```python
from build123d import *

# Parameters (mm, degrees)
RESSALTO_EXTRUS_O1_DEPTH        = 7.5
FURO_ROSCADO_DE_M31_D           = 2.5
FURO_ROSCADO_DE_M31_DEPTH       = 7.5
FURO_ROSCADO_DE_M31_CSINK_D     = 3.05
FURO_ROSCADO_DE_M31_CSINK_ANGLE = 90
FURO_ROSCADO_DE_M31_TIP         = 0.751075774
CHANFRO1_SIZE                   = 5


with BuildPart() as part:
    # Esboço1 → Ressalto-extrusão1 (new, symmetric)
    with BuildSketch(Plane(origin=(0, 0, 0), x_dir=(1, 0, 0), z_dir=(0, 1, 0))):
        Polygon((3.666174209, 6.35), (-3.666174209, 6.35), (-8, 6.35), (-8, -6.35), (8, -6.35), (8, 6.35), align=None)
    extrude(amount=RESSALTO_EXTRUS_O1_DEPTH, both=True)

    # Esboço5 → Furo roscado de M81 (revolve, cut)
    with BuildSketch(Plane(origin=(0, 7.5, 0), x_dir=(0, 0, 1), z_dir=(1, 0, 0))):
        Polygon((0, 0), (0, 15), (4, 15), (3.4, 14.4), (3.4, 0.6), (4, 0), align=None)
    revolve(axis=Axis((0, 13.85, 0), (0, -1, 0)), mode=Mode.SUBTRACT)

    # Furo roscado de M31
    with Locations(Plane(origin=(0, 0, -6.35), x_dir=(-1, 0, 0), z_dir=(0, 0, -1))):
        with Locations((-6, 0), (6, 0)):
            CounterSinkHole(FURO_ROSCADO_DE_M31_D / 2, FURO_ROSCADO_DE_M31_CSINK_D / 2, depth=FURO_ROSCADO_DE_M31_DEPTH, counter_sink_angle=FURO_ROSCADO_DE_M31_CSINK_ANGLE)
            with Locations((0, 0, -(FURO_ROSCADO_DE_M31_DEPTH + FURO_ROSCADO_DE_M31_TIP / 2))):  # 118° drill point
                Cone(0, FURO_ROSCADO_DE_M31_D / 2, FURO_ROSCADO_DE_M31_TIP, mode=Mode.SUBTRACT)

    # Chanfro1
    chanfro1_edges = [part.edges().sort_by_distance(p)[0] for p in [
        (8, 0, 6.35),
        (-8, 0, 6.35),
    ]]
    chamfer(chanfro1_edges, length=CHANFRO1_SIZE)


solid = part.part
```
Here's how the part is built. I have some questions about the finished solid (model axes, mm). A direction names the side the tool comes from. Round coordinates to 2 decimals unless told otherwise and drop trailing zeros. Order: outer loops, then holes, each group sorted by start corner. A loop starts at its lowest first (then second) coordinate and runs counter-clockwise, first axis right, second up. Notation, with made-up numbers: (-24.75, 79.5) -> (-3.75, 79.5) arc R26 ccw to (-3.75, 116.5) -> close; hole circle Ø3 at (-24.75, 7.5). An arc over 180 degrees is marked (long way). Use a Markdown table: item, result. Add a question column.
(1) For pin 1 Ø3 at (x, y) = (-6, 0) entering from -Z (3 decimals); pin 2 Ø2 at (x, y) = (6, 0) entering from +Z, each with a flat end and sliding along its axis, tell me the tip position at first contact or that it passes through.
(2) I need wall thicknesses on line 1 along Z through (x, y) = (0, -3); line 2 along X through (y, z) = (1.75, 0); line 3 along X through (y, z) = (0, -0.75). Which ranges of each line are inside material? Lowest first, please.
(3) For faces 1 (the face through (-7.25, 0.05, -2.41)), 2 (the face through (-0.1, -7.5, -4.3)), which set-ups out of +Z, -Z, +X, -X, +Y, -Y let a thin tool reach every point of the face, with its end or its side?
(4) Suppose I cut it at C-C, the plane x = 0. Please give me the cut outline in (y, z), and give its area (3 significant figures).
(5) Suppose I cut it at A-A, the plane z = 0. Please give me the cut outline in (x, y).
(6) If we mould it in two halves opening along Z, with no side actions, what happens to faces 3 (the face through (-0.1, 7.5, -4.3)), 4 (the face through (-5.78, 0.01, 1.77)), 5 (the face through (3.32, 0.1, -0.74)), 6 (the face through (-5.465, -0.105, 3.885))? For each: released by +Z, released by -Z, zero draft, split by the parting line, or undercut.
(7) Suppose I cut it at D-D, the plane z = -4.5. Please give me the cut outline in (x, y), and give its area (3 significant figures).
(8) Suppose I cut it at B-B, the plane y = -6. Please give me the cut outline in (x, z), and give its area (3 significant figures).
Verdict:
| question | item | result |
|---|---|---|
| 1 | pin 1 | z = -6.325 |
| 1 | pin 2 | z = 4.35 |
| 2 | line 1 | -6.35 to -3.4, 3.4 to 6.35 |
| 2 | line 2 | -8 to -3.4, 3.4 to 8 |
| 2 | line 3 | -8 to -7.25, -4.75 to -3.32, 3.32 to 4.75, 7.25 to 8 |
| 3 | face 1 | -Z |
| 3 | face 2 | +Z, -Z, +X, -X, -Y |
| 4 | outline | (-7.5, -6.35) -> (7.5, -6.35) -> (7.5, -4) -> (6.9, -3.4) -> (-6.9, -3.4) -> (-7.5, -4) -> close; (-7.5, 4) -> (-6.9, 3.4) -> (6.9, 3.4) -> (7.5, 4) -> (7.5, 6.35) -> (-7.5, 6.35) -> close |
| 4 | area | 87.8 mm2 |
| 5 | outline | (-8, -7.5) -> (-4, -7.5) -> (-3.4, -6.9) -> (-3.4, 6.9) -> (-4, 7.5) -> (-8, 7.5) -> close; (3.4, -6.9) -> (4, -7.5) -> (8, -7.5) -> (8, 7.5) -> (4, 7.5) -> (3.4, 6.9) -> close; hole circle Ø2.5 at (-6, 0); hole circle Ø2.5 at (6, 0) |
| 6 | face 3 | zero draft |
| 6 | face 4 | released by -Z |
| 6 | face 5 | undercut |
| 6 | face 6 | released by +Z |
| 7 | outline | (-8, -7.5) -> (8, -7.5) -> (8, 7.5) -> (-8, 7.5) -> close; hole circle Ø2.5 at (-6, 0); hole circle Ø2.5 at (6, 0) |
| 7 | area | 230 mm2 |
| 8 | outline | (-8, -6.35) -> (8, -6.35) -> (8, 1.35) -> (3, 6.35) -> (-3, 6.35) -> (-8, 1.35) -> close; hole circle Ø6.8 at (0, 0) |
| 8 | area | 142 mm2 |
